Read the model definition and answer for the solid it produces. Units are mm, in the model's axes. A direction names the side the tool comes from. Coordinates: 2 decimals unless noted, no trailing zeros. Loops run counter-clockwise (first coordinate to the right, second up) from the corner with the lowest first, then second, coordinate; pieces in that order, holes last. Notation, with made-up numbers: (48, -15.5) - (78, -15.5) arc R25 ccw to (78, 18.5) - close; hole circle Ø5 at (75.25, 50.5). An arc over 180 degrees is marked (long way). One line per question, with ' | ' between items. Start each with the question number.
```python
from build123d import *

# Parameters (mm, degrees)
SKETCH1_W               = 750
SKETCH1_H               = 450
BOSS_EXTRUDE1_DEPTH     = 310
SKETCH8_W               = 750
SKETCH8_H               = 300
CUT_EXTRUDE1_DEPTH      = 445
SKETCH15_W              = 5
SKETCH15_H              = 250
BOSS_EXTRUDE8_DEPTH     = 100
CUT_EXTRUDE2_DEPTH      = 537.050370768
CUT_EXTRUDE2_DEPTH_BACK = 10
SKETCH16_R              = 5
SKETCH16_W              = 750
SKETCH16_H              = 250
SKETCH18_W              = 5
SKETCH18_H              = 5
CUT_EXTRUDE3_DEPTH      = 537.050370768
SKETCH10_R              = 2.5
CUT_EXTRUDE4_DEPTH      = 534.174455502


with BuildPart() as part:
    # Sketch1 → Boss-Extrude1 (new body)
    with BuildSketch(Plane(origin=(0, 0, 0), x_dir=(1, 0, 0), z_dir=(0, 1, 0))):
        Rectangle(SKETCH1_W, SKETCH1_H)
    extrude(amount=BOSS_EXTRUDE1_DEPTH)

    # Sketch8 → Cut-Extrude1 (cut)
    with BuildSketch(Plane.XY.offset(225)):
        with Locations((0, 155)):
            Rectangle(SKETCH8_W, SKETCH8_H)
    extrude(amount=-CUT_EXTRUDE1_DEPTH, mode=Mode.SUBTRACT)

    # Sketch15 → Boss-Extrude8 (add)
    with BuildSketch(Plane(origin=(0, 5, 0), x_dir=(1, 0, 0), z_dir=(0, 1, 0))):
        with Locations((172.5, 95)):
            Rectangle(SKETCH15_W, SKETCH15_H)
    extrude(amount=BOSS_EXTRUDE8_DEPTH)

    # Sketch16 → Cut-Extrude2 (cut, two sides: drawn at the far end of the back side and taken through both)
    with BuildSketch(Plane(origin=(0, 310, 0), x_dir=(1, 0, 0), z_dir=(0, 1, 0)).offset(-CUT_EXTRUDE2_DEPTH_BACK)):
        with Locations(Location((275, 75, 0), (0, 0, 90))):
            Circle(SKETCH16_R)
        with Locations(Location((-225, 75, 0), (0, 0, 90))):
            Circle(SKETCH16_R)
        with Locations((0, -100)):
            Rectangle(SKETCH16_W, SKETCH16_H)
    extrude(amount=CUT_EXTRUDE2_DEPTH + CUT_EXTRUDE2_DEPTH_BACK, mode=Mode.SUBTRACT)

    # Sketch18 → Cut-Extrude3 (cut, through all)
    with BuildSketch(Plane(origin=(0, 310, 0), x_dir=(1, 0, 0), z_dir=(0, 1, 0))):
        with Locations((-362.5, 37.5)):
            Rectangle(SKETCH18_W, SKETCH18_H)
        with Locations((362.5, 37.5)):
            Rectangle(SKETCH18_W, SKETCH18_H)
    extrude(amount=-CUT_EXTRUDE3_DEPTH, mode=Mode.SUBTRACT)

    # Sketch10 → Cut-Extrude4 (cut, through all)
    with BuildSketch(Plane(origin=(0, 5, 0), x_dir=(1, 0, 0), z_dir=(0, 1, 0))):
        with Locations(Location((-250, 0, 0), (0, 0, 270))):
            Circle(SKETCH10_R)
        with Locations(Location((-150, 0, 0), (0, 0, 270))):
            Circle(SKETCH10_R)
    extrude(amount=-CUT_EXTRUDE4_DEPTH, mode=Mode.SUBTRACT)


solid = part.part
```
1) The part is cut by section A-A on z = -181. Write down the section's boundary in (x, y), and give its area (3 significant figures).
2) Find the intervals of material crossed by line 1 along X through (y, z) = (307.9, -75); line 2 along X through (y, z) = (3.35, 0); line 3 along Y through (x, z) = (-142, -160), in increasing order. Write a range as from..to.
3) Which of the six approach directions +Z, -Z, +X, -X, +Y, -Y give full straight-line access (tool end or side, diameter ignored) to faces 1 (the flat face through (-5, 5, 6)), 2 (the flat face through (175, 54, -93)), 3 (the flat face through (-5, 310, -126)), 4 (the flat face through (-5, 305, -121))?
4) The mould has two halves that part along Y. Classify faces 5 (the flat face through (170, 54, -93)), 6 (the flat face through (-5, 0, -3)), 7 (the flat face through (-5, 153, -225)), 8 (the flat face through (-5, 157, -220)): released by +Y, released by -Y, zero draft, split by the parting line, or undercut.
5) The part is cut by section C-C on z = 12. Write down the section's boundary in (x, y), and give its area (3 significant figures).
6) The part is cut by section D-D on z = 191. Write down the section's boundary in (x, y).
7) The part is cut by section B-B on y = 80.5. Write down the section's boundary in (x, z).
8) Given pin 1 Ø1.5 at (x, y) = (-362, 306.5) entering from +Z; pin 2 Ø16 at (x, z) = (275, -75) entering from +Y; pin 3 Ø8 at (y, z) = (102.5, -81) entering from +X; pin 4 Ø1.5 at (x, y) = (172.5, 31.5) entering from +Z, each flat-ended and moving along its own axis, determine where each tip first touches the part or whether it passes through.
Answer below:
1) outline: (-375, 0) - (375, 0) - (375, 5) - (175, 5) - (175, 105) - (170, 105) - (170, 5) - (-375, 5) - close; (-375, 305) - (375, 305) - (375, 310) - (-375, 310) - close | area: 8,000 mm2
2) line 1: -375..-230, -220..270, 280..375 | line 2: -375..-252.5, -247.5..-152.5, -147.5..375 | line 3: 0..5, 305..310
3) face 1: +Z | face 2: +Z, +X | face 3: +Z, -Z, +X, -X, +Y | face 4: +Z, +X, -X
4) face 5: undercut | face 6: released by -Y | face 7: zero draft | face 8: undercut
5) outline: (-375, 0) - (375, 0) - (375, 5) - (175, 5) - (175, 105) - (170, 105) - (170, 5) - (-375, 5) - close | area: 4,250 mm2
6) outline: (-375, 0) - (375, 0) - (375, 5) - (-375, 5) - close
7) outline: (-375, -225) - (375, -225) - (375, -220) - (175, -220) - (175, 30) - (170, 30) - (170, -220) - (-375, -220) - close
8) pin 1: z = -25 | pin 2: y = 310 | pin 3: x = 175 | pin 4: z = 30
